```python
from build123d import *

# Parameters (mm, degrees)
F0_R      = 44.45
F1_DEPTH  = 12.7
F2_R      = 42.8625
F4_DEPTH  = 12.7
F3_R      = 42.8625
F5_DEPTH  = 9.525
F8_R      = 3.175
F9_DEPTH  = 63.5
F7_R      = 3.175
F10_DEPTH = 63.5
F15_R     = 1.5875
F16_DEPTH = 76.2
F17_R     = 1.5875
F18_DEPTH = 63.5
F6_R      = 38.1
F19_DEPTH = 12.7


with BuildPart() as f1:
    # F0 (on Front) → F1 (new body, symmetric)
    with BuildSketch(Plane.XZ):
        Circle(F0_R)
    extrude(amount=F1_DEPTH, both=True)

    # F2 (on Front) → F4 (cut, symmetric)
    with BuildSketch(Plane.XZ):
        Circle(F2_R)
    extrude(amount=F4_DEPTH, both=True, mode=Mode.SUBTRACT)

    # F3 (on Front) → F5 (join, symmetric)
    with BuildSketch(Plane.XZ):
        Circle(F3_R)
    extrude(amount=F5_DEPTH, both=True)

    # F8 (on Top) → F9 (join)
    with BuildSketch(Plane.XY):
        with Locations((25.4, 0)):
            Circle(F8_R)
    extrude(amount=-F9_DEPTH)

    # F7 (on Top) → F10 (join)
    with BuildSketch(Plane.XY):
        with Locations((-25.4, 0)):
            Circle(F7_R)
    extrude(amount=-F10_DEPTH)

    # F11 (on Front) → F12 (revolve)
    with BuildSketch(Plane.XZ):
        Polygon((28.479918, -55.88), (28.480154, -62.23), (29.749918, -55.88), align=None)
    revolve(axis=Axis((25.4, 0, -63.5), (0, 0, 1)))

    # F13 (on Front) → F14 (revolve)
    with BuildSketch(Plane.XZ):
        Polygon((-22.225006, -55.88), (-22.225006, -62.23), (-20.955006, -55.88), align=None)
    revolve(axis=Axis((-25.4, 0, -63.5), (0, 0, 1)))

    # F15 (on face) → F16 (cut)
    with BuildSketch(Plane(origin=(0, 0, -63.5), x_dir=(1, 0, 0), z_dir=(0, 0, -1))):
        with Locations((25.4, 0)):
            Circle(F15_R)
    extrude(amount=-F16_DEPTH, mode=Mode.SUBTRACT)

    # F17 (on face) → F18 (cut)
    with BuildSketch(Plane(origin=(0, 0, -63.5), x_dir=(1, 0, 0), z_dir=(0, 0, -1))):
        with Locations((-25.4, 0)):
            Circle(F17_R)
    extrude(amount=-F18_DEPTH, mode=Mode.SUBTRACT)

    # F6 (on Front) → F19 (cut, symmetric)
    with BuildSketch(Plane.XZ):
        Circle(F6_R)
    extrude(amount=F19_DEPTH, both=True, mode=Mode.SUBTRACT)


solid = f1.part
```
Geometry: final body of the model. Coordinates: model frame, mm. A direction names the side the tool comes from. Give positions to 0.01 mm unless a question says otherwise; leave off trailing zeros. Use CSV: the item, a comma, the result in double quotes.
(1) Cut plane C-C (x = 25.4). Count the separate pieces of the cut face and the enclosed holes in it, plus the area to 3 significant figures.
From the geometry:
separate pieces,"3"
enclosed holes,"0"
area,"400 mm^2"
(2) Pull-direction query (X, two-part tool) for faces 4 (the face through (28.872, 1.093, -59.43)), 5 (the face through (-23.3, -12.7, 36.4)); classes: released by +X, released by -X, zero draft, split by the parting line, or undercut.
From the geometry:
face 4,"undercut"
face 5,"zero draft"
(3) Ray query, line 1 along Z through (x, y) = (0, -10.95); line 2 along X through (y, z) = (0, -40.5) (1 decimal); line 3 along Z through (x, y) = (-1, 7). Return the intervals inside material, ascending. Write a range as [from, to].
From the geometry:
line 1,"[-44.45, -42.86], [42.86, 44.45]"
line 2,"[-28.6, -27], [-23.8, -22.2], [-18.3, 18.3], [22.2, 23.8], [27, 28.6]"
line 3,"[-44.44, -38.09], [38.09, 44.44]"
(4) Access query for faces 1 (the face through (23.043, -11.135, 36.142)), 2 (the face through (23, -3, -55.88)), 3 (the face through (-22.37, 0.95, -62.86)). Directions: +Z, -Z, +X, -X, +Y, -Y. A direction counts if a zero-diameter tool reaches every point of the face in a straight line with its end or side. Return the directions, or none.
From the geometry:
face 1,"-Y"
face 2,"none"
face 3,"-Z"
(5) First-contact query: P1, Ø5, axis at x = 29.5, y = 3, coming from the +Z side; P2, Ø12, axis at y = 0.5, z = -2.5, coming from the +X side; P3, Ø10, axis at x = -24.5, y = -2, coming from the +Z side; P4, Ø12, axis at x = 26.5, y = 3, coming from the +Z side. Flat tips, straight axial feed; report the tip coordinate or a pass-through.
From the geometry:
P1,"z = 35.31"
P2,"x = 44.45"
P3,"z = 39.94"
P4,"z = 39.44"
